Check sheet for the modelled part. Datum: model origin and axes. Units: mm. Give positions to 0.01 mm unless a question says otherwise; leave off trailing zeros. Loops run counter-clockwise (first coordinate to the right, second up) from the corner with the lowest first, then second, coordinate; pieces in that order, holes last. Notation, with made-up numbers: (-13, -37) - (24, -37) arc R24 ccw to (24, -27) - close; hole circle Ø6 at (2, -27). An arc over 180 degrees is marked (long way). Use CSV: the item, a comma, the result in double quotes.
from build123d import *

# Parameters (mm, degrees)
F0_R           = 5
F0_R_2         = 6.0157611954
F0_R_3         = 5.450221674
F0_R_4         = 4
F0_R_5         = 2
F0_R_6         = 3.4791274017
F0_R_7         = 5.4671936668
F0_R_8         = 4.2465190739
F0_R_9         = 3.1434156929
F0_R_10        = 6.9718270278
F0_R_11        = 3.5055270759
F1_DEPTH       = 6
F2_D           = 5.5
F2_CSINK_D     = 8.96
F2_CSINK_ANGLE = 90
F3_D           = 4.5
F3_CSINK_D     = 8.96
F3_CSINK_ANGLE = 90
F4_D           = 6.6
F6_D           = 2.7
F6_DEPTH       = 12
F6_TIP         = 0.8111618357
F8_D           = 2.7
F8_DEPTH       = 12
F8_TIP         = 0.8111618357
F9_R           = 5


with BuildPart() as f1:
    # F0 (on Front) → F1 (new body)
    with BuildSketch(Plane.XZ):
        with BuildLine():
            ThreePointArc((-96.4640628632, -18.4166666667), (-78.1054529592, -41.7057843836), (-49.7843771792, -50.5))
            Line((-49.7843771792, -50.5), (115, -50.5))
            Line((115, -50.5), (115, 50.5))
            Line((115, 50.5), (-49.7843771792, 50.5))
            ThreePointArc((-49.7843771792, 50.5), (-78.1054529592, 41.7057843836), (-96.4640628632, 18.4166666667))
            ThreePointArc((-96.4640628632, 18.4166666667), (-100.135784844, 13.7588431233), (-105.8, 12))
            Line((-105.8, 12), (-115, 12))
            ThreePointArc((-115, 12), (-127, 0), (-115, -12))
            Line((-115, -12), (-105.8, -12))
            ThreePointArc((-105.8, -12), (-100.135784844, -13.7588431233), (-96.4640628632, -18.4166666667))
        make_face()
        with Locations((-115, 0)):
            Circle(F0_R, mode=Mode.SUBTRACT)
        with Locations((-53.41, -15.6)):
            Circle(F0_R_2, mode=Mode.SUBTRACT)
        with Locations((-24.28, -23.2)):
            Circle(F0_R_3, mode=Mode.SUBTRACT)
        with Locations((-19.15, -9.1)):
            Circle(F0_R_4, mode=Mode.SUBTRACT)
        with Locations((48, -39.8021750152)):
            Circle(F0_R_5, mode=Mode.SUBTRACT)
        with Locations((13, -20)):
            Circle(F0_R_5, mode=Mode.SUBTRACT)
        with BuildLine():
            ThreePointArc((32.1548065788, -12.2036816348), (41.5542210876, 18.9328268944), (68, 0))
            ThreePointArc((68, 0), (59.1108283975, -16.6297772782), (40.3450507679, -18.4770601626))
            ThreePointArc((40.3450507679, -18.4770601626), (41.2075439734, -20.9229943569), (41.5, -23.5))
            ThreePointArc((41.5, -23.5), (21.1391231908, -30.8304066853), (32.1548065788, -12.2036816348))
        make_face(mode=Mode.SUBTRACT)
        with Locations((81, -18.5)):
            Circle(F0_R_4, mode=Mode.SUBTRACT)
        with Locations((103, -23.5)):
            Circle(F0_R_6, mode=Mode.SUBTRACT)
        with Locations((-48.28, 1.52)):
            Circle(F0_R_4, mode=Mode.SUBTRACT)
        with Locations((-14.02, 5)):
            Circle(F0_R_7, mode=Mode.SUBTRACT)
        with Locations((-43.15, 15.6)):
            Circle(F0_R_8, mode=Mode.SUBTRACT)
        with Locations((-9.25, 44.8)):
            Circle(F0_R_9, mode=Mode.SUBTRACT)
        with Locations((30, 23.5)):
            Circle(F0_R_10, mode=Mode.SUBTRACT)
        with Locations((81, 18.5)):
            Circle(F0_R_4, mode=Mode.SUBTRACT)
        with Locations((103, 23.5)):
            Circle(F0_R_11, mode=Mode.SUBTRACT)
        with BuildLine():
            ThreePointArc((17.1984440191, 41.7107700429), (24.0572213428, 43.8278941274), (28.2477691357, 38))
            ThreePointArc((28.2477691357, 38), (25.1621574991, 32.669122324), (19.0027060342, 32.6894599677))
            ThreePointArc((19.0027060342, 32.6894599677), (5.9710481835, 31.4127376868), (10.8695627244, 43.5559943098))
            ThreePointArc((10.8695627244, 43.5559943098), (12.5588245291, 47.3626903964), (15.8416828069, 44.8))
            ThreePointArc((15.8416828069, 44.8), (15.6633729559, 43.845913142), (15.152514728, 43.0206253094))
            ThreePointArc((15.152514728, 43.0206253094), (16.2277672329, 42.4473687323), (17.1984440191, 41.7107700429))
        make_face(mode=Mode.SUBTRACT)
        with Locations((-43.15, 15.6)):
            Circle(F0_R_8)
        with Locations((-53.41, -15.6)):
            Circle(F0_R_2)
        with Locations((-14.02, 5)):
            Circle(F0_R_7)
        with Locations((-24.28, -23.2)):
            Circle(F0_R_3)
        with BuildLine():
            ThreePointArc((19.0027060342, 32.6894599677), (16.071616387, 36.7943232774), (17.1984440191, 41.7107700429))
            ThreePointArc((17.1984440191, 41.7107700429), (16.2277672329, 42.4473687323), (15.152514728, 43.0206253094))
            ThreePointArc((15.152514728, 43.0206253094), (12.8723395742, 42.1787165934), (10.8695627244, 43.5559943098))
            ThreePointArc((10.8695627244, 43.5559943098), (5.9710481835, 31.4127376868), (19.0027060342, 32.6894599677))
        make_face()
        with BuildLine():
            ThreePointArc((19.0027060342, 32.6894599677), (25.1621574991, 32.669122324), (28.2477691357, 38))
            ThreePointArc((28.2477691357, 38), (24.0572213428, 43.8278941274), (17.1984440191, 41.7107700429))
            ThreePointArc((17.1984440191, 41.7107700429), (19.0870694567, 39.1285597815), (19.7555225752, 36))
            ThreePointArc((19.7555225752, 36), (19.5649463419, 34.3024717933), (19.0027060342, 32.6894599677))
        make_face()
        with Locations((30, 23.5)):
            Circle(F0_R_10)
        with BuildLine():
            ThreePointArc((40.3450507679, -18.4770601626), (35.8384624442, -15.87756292), (32.1548065788, -12.2036816348))
            ThreePointArc((32.1548065788, -12.2036816348), (21.1391231908, -30.8304066853), (41.5, -23.5))
            ThreePointArc((41.5, -23.5), (41.2075439734, -20.9229943569), (40.3450507679, -18.4770601626))
        make_face()
        with Locations((103, 23.5)):
            Circle(F0_R_11)
        with Locations((103, -23.5)):
            Circle(F0_R_6)
        with BuildLine():
            ThreePointArc((10.8695627244, 43.5559943098), (13.0495507108, 43.596405686), (15.152514728, 43.0206253094))
            ThreePointArc((15.152514728, 43.0206253094), (15.6633729559, 43.845913142), (15.8416828069, 44.8))
            ThreePointArc((15.8416828069, 44.8), (12.5588245291, 47.3626903964), (10.8695627244, 43.5559943098))
        make_face()
        with BuildLine():
            ThreePointArc((10.8695627244, 43.5559943098), (12.8723395742, 42.1787165934), (15.152514728, 43.0206253094))
            ThreePointArc((15.152514728, 43.0206253094), (13.0495507108, 43.596405686), (10.8695627244, 43.5559943098))
        make_face()
        with Locations((-9.25, 44.8)):
            Circle(F0_R_9)
        with BuildLine():
            ThreePointArc((19.7555225752, 36), (19.0870694567, 39.1285597815), (17.1984440191, 41.7107700429))
            ThreePointArc((17.1984440191, 41.7107700429), (16.071616387, 36.7943232774), (19.0027060342, 32.6894599677))
            ThreePointArc((19.0027060342, 32.6894599677), (19.5649463419, 34.3024717933), (19.7555225752, 36))
        make_face()
    extrude(amount=F1_DEPTH)

    # F2 (through all)
    with Locations(Plane(origin=(0, 0, 0), x_dir=(1, 0, 0), z_dir=(0, 1, 0))):
        with Locations((-43.15, -15.6), (-53.41, 15.6), (-14.02, -5), (-24.28, 23.2), (30, 23.5), (30, -23.5), (103, -23.5), (103, 23.5)):
            CounterSinkHole(F2_D / 2, F2_CSINK_D / 2, counter_sink_angle=F2_CSINK_ANGLE)

    # F3 (through all)
    with Locations(Plane(origin=(0, 0, 0), x_dir=(1, 0, 0), z_dir=(0, 1, 0))):
        with Locations((22.1, -38), (12.1, -36)):
            CounterSinkHole(F3_D / 2, F3_CSINK_D / 2, counter_sink_angle=F3_CSINK_ANGLE)

    # F4 (through all)
    with Locations(Plane(origin=(0, 0, 0), x_dir=(1, 0, 0), z_dir=(0, 1, 0))):
        with Locations((-9.25, -44.8), (13.2, -44.8)):
            Hole(F4_D / 2)

    # F6
    with Locations(Plane(origin=(0, 0, -50.5), x_dir=(1, 0, 0), z_dir=(0, 0, -1))):
        with Locations((60, 3), (-25, 3)):
            Hole(F6_D / 2, depth=F6_DEPTH)
            with Locations((0, 0, -(F6_DEPTH + F6_TIP / 2))):  # 118° drill point
                Cone(0, F6_D / 2, F6_TIP, mode=Mode.SUBTRACT)

    # F8
    with Locations(Plane.XY.offset(50.5)):
        with Locations((-25, -3), (60, -3)):
            Hole(F8_D / 2, depth=F8_DEPTH)
            with Locations((0, 0, -(F8_DEPTH + F8_TIP / 2))):  # 118° drill point
                Cone(0, F8_D / 2, F8_TIP, mode=Mode.SUBTRACT)

    # F9
    f9_edges = [f1.edges().sort_by_distance(p)[0] for p in [
        (115, -3, 50.5),
        (115, -3, -50.5),
    ]]
    fillet(f9_edges, radius=F9_R)


solid = f1.part
1. Release check for a two-part mould opening along X. For faces 1 (the face through (12.611, -2.122, 38.302)), 2 (the face through (113.5, -3.04, -49.07)), 3 (the face through (-127, -3, 0)) record: released by +X, released by -X, zero draft, split by the parting line, or undercut.
Completed:
face 1,"undercut"
face 2,"released by +X"
face 3,"released by -X"
2. Scan lines: line 1 along Z through (x, y) = (103, -4.45); line 2 along X through (y, z) = (-2.95, 44.8); line 3 along X through (y, z) = (-4.3, -13.5). Record each from-to range of solid material in increasing order.
Completed:
line 1,"z = -50.5 to -26.25, -20.75 to 20.75, 26.25 to 50.5"
line 2,"x = -72.97 to -26.35, -23.65 to -12.55, -5.95 to 9.9, 16.5 to 58.65, 61.35 to 115"
line 3,"x = -100.53 to -55.19, -51.63 to 33.24, 62.76 to 115"
3. Sectioned sample at A-A, the plane x = 81. Record the boundary of the cut face in (y, z), and give its area (3 significant figures).
Completed:
outline,"(-6, -50.5) - (0, -50.5) - (0, -22.5) - (-6, -22.5) - close; (-6, -14.5) - (0, -14.5) - (0, 14.5) - (-6, 14.5) - close; (-6, 22.5) - (0, 22.5) - (0, 50.5) - (-6, 50.5) - close"
area,"510 mm²"
4. Go/stop test with flat-tipped pins: pin 1 Ø6 at (x, z) = (-9.25, 44.8) entering from +Y; pin 2 Ø1 at (y, z) = (-3.5, -35.5) entering from -X; pin 3 Ø7 at (x, z) = (12.1, 36) entering from +Y; pin 4 Ø3 at (x, y) = (-112.5, -3) entering from +Z. Record where each tip stops, or that it passes through.
Completed:
pin 1,"passes through"
pin 2,"stops at x = -85.97"
pin 3,"stops at y = -0.98"
pin 4,"stops at z = 12"
